from build123d import *

# Parameters (mm, degrees)
F1_DEPTH       = 15
F3_D           = 3.1
F3_DEPTH       = 15
F3_TIP         = 0.9313339595
F4_W           = 15
F4_H           = 3
F5_DEPTH       = 15
F8_D           = 3.1
F8_DEPTH       = 3
F8_TIP         = 0.9313339595
F8_ON_F7_D     = 3.1
F8_ON_F7_DEPTH = 3
F8_ON_F7_TIP   = 0.9313339595


with BuildPart() as f1:
    # F0 (on Front) → F1 (new body)
    with BuildSketch(Plane.XZ):
        with BuildLine():
            Line((-7.4164065372, 11.0490259535), (-19.4164065372, 11.0490259535))
            Line((-19.4164065372, 11.0490259535), (-19.4164065372, 8.0490259535))
            Line((-19.4164065372, 8.0490259535), (-19.4164065372, -10.7509740465))
            Line((-19.4164065372, -10.7509740465), (21.5835934628, -10.7509740465))
            Line((21.5835934628, -10.7509740465), (21.5835934628, 8.0490259535))
            Line((21.5835934628, 8.0490259535), (21.5835934628, 15.5490259535))
            Line((21.5835934628, 15.5490259535), (11.9898709467, 15.5490259535))
            ThreePointArc((11.9898709467, 15.5490259535), (1.0835934628, 23.3204583115), (-9.8226840211, 15.5490259535))
            Line((-9.8226840211, 15.5490259535), (-19.4164065372, 15.5490259535))
            Line((-19.4164065372, 15.5490259535), (-19.4164065372, 12.5490259535))
            Line((-19.4164065372, 12.5490259535), (-7.4164065372, 12.5490259535))
            ThreePointArc((-7.4164065372, 12.5490259535), (1.0835934628, 20.29968098), (9.5835934628, 12.5490259535))
            Line((9.5835934628, 12.5490259535), (15.1835934628, 12.5490259535))
            Line((15.1835934628, 12.5490259535), (15.1835934628, 11.0490259535))
            Line((15.1835934628, 11.0490259535), (12.5835934628, 11.0490259535))
            Line((12.5835934628, 11.0490259535), (9.5835934628, 11.0490259535))
            ThreePointArc((9.5835934628, 11.0490259535), (1.0835934628, 3.294835898), (-7.4164065372, 11.0490259535))
        make_face()
    extrude(amount=F1_DEPTH)

    # F3
    with Locations(Plane.XY.offset(15.5490259535)):
        with Locations((-14.6195452792, -7.5)):
            Hole(F3_D / 2, depth=F3_DEPTH)
            with Locations((0, 0, -(F3_DEPTH + F3_TIP / 2))):  # 118° drill point
                Cone(0, F3_D / 2, F3_TIP, mode=Mode.SUBTRACT)

    # F4 (on face) → F5 (join)
    with BuildSketch(Plane.XZ.offset(15)):
        with Locations((13.5835934628, -9.2509740465)):
            Rectangle(F4_W, F4_H)
        with Locations((-11.4164065372, -9.2509740465)):
            Rectangle(F4_W, F4_H)
    extrude(amount=F5_DEPTH)

    # F8
    with Locations(Plane.XY.offset(-7.7509740465)):
        with Locations((-11.4164065372, -22.5)):
            Hole(F8_D / 2, depth=F8_DEPTH)
            with Locations((0, 0, -(F8_DEPTH + F8_TIP / 2))):  # 118° drill point
                Cone(0, F8_D / 2, F8_TIP, mode=Mode.SUBTRACT)

    # F8 on F7
    with Locations(Plane.XY.offset(-7.7509740465)):
        with Locations((13.5835934628, -22.5)):
            Hole(F8_ON_F7_D / 2, depth=F8_ON_F7_DEPTH)
            with Locations((0, 0, -(F8_ON_F7_DEPTH + F8_ON_F7_TIP / 2))):  # 118° drill point
                Cone(0, F8_ON_F7_D / 2, F8_ON_F7_TIP, mode=Mode.SUBTRACT)


solid = f1.part
Here's how the part is built. I have some questions about the finished solid (model axes, mm). A direction names the side the tool comes from. Give positions to 0.01 mm unless a question says otherwise; leave off trailing zeros. Order: outer loops, then holes, each group sorted by start corner. A loop starts at its lowest first (then second) coordinate and runs counter-clockwise, first axis right, second up. Notation, with made-up numbers: M 55.25,-9.5 L 108.25,-9.5 A21 cw 108.25,18.5 Z; hole C 50,1.5 d9. An arc over 180 degrees is marked long. Answer as a JSON object with one key per item and string values. Group by question number.
1) Suppose I cut it at C-C, the plane x = -5. Write out the boundary of the cut face in (y, z).
2) Suppose I cut it at D-D, the plane y = -26.75. Write out the boundary of the cut face in (x, z), plus the area to 3 significant figures.
3) I'm going to push flat-ended pins straight in: pin 1 Ø10 at (y, z) = (-15.5, -2.5) entering from -X; pin 2 Ø8 at (x, y) = (-5.5, -9.5) entering from +Z; pin 3 Ø3.5 at (y, z) = (-23.5, -9) entering from +X; pin 4 Ø13 at (x, y) = (-12.5, -4) entering from +Z. Where does each tip first touch, or does it pass through?
4) We'd pull the mould along Y, two halves only. Please class faces 5 (the conical face through (-14.89, -7.49, -0.22)), 6 (the flat face through (0.8, -14.8, -10.751)): pulls with the +Y half, pulls with the -Y half, needs draft (parallel to the pull), parting line crosses it, or undercut.
5) Suppose I cut it at A-A, the plane z = 10. Write out the boundary of the cut face in (x, y).
6) Suppose I cut it at B-B, the plane y = -22.5. Write out the boundary of the cut face in (x, z).
7) Please list where these lines run through material, in increasing order: L1, parallel to X at y = -22.5, z = -9.45; L2, parallel to X at y = -6.25, z = 13; L3, parallel to X at y = -7.5, z = 7.75. Write a range as [from, to].
8) On a 3-axis mill with a long thin cutter (end or side, diameter ignored), from which of +Z, -Z, +X, -X, +Y, -Y can I reach the whole of each face in a straight line? I mean faces 1 (the flat face through (-18.916, -22, -9)), 2 (the flat face through (-11.5, -20.7, -7.751)), 3 (the flat face through (-3.916, -22, -9)), 4 (the flat face through (17, -7, 15.549)). Say none if no direction works.
Results found:
{
 "1": {"outline": "M -30,-10.75 L 0,-10.75 L 0,5.84 L -15,5.84 L -15,-7.75 L -30,-7.75 Z; M -15,17.75 L 0,17.75 L 0,21.59 L -15,21.59 Z"},
 "2": {"outline": "M -18.92,-10.75 L -3.92,-10.75 L -3.92,-7.75 L -18.92,-7.75 Z; M 6.08,-10.75 L 21.08,-10.75 L 21.08,-7.75 L 6.08,-7.75 Z", "area": "90.0 mm²"},
 "3": {"pin 1": "x = -19.42", "pin 2": "z = 23.03", "pin 3": "x = 21.08", "pin 4": "z = 20.89"},
 "4": {"face 5": "undercut", "face 6": "needs draft"},
 "5": {"outline": "M -19.42,-15 L -7.25,-15 L -7.25,0 L -19.42,0 Z; M 9.42,-15 L 21.58,-15 L 21.58,0 L 9.42,0 Z; hole C -14.62,-7.5 d3.1"},
 "6": {"outline": "M -18.92,-10.75 L -12.97,-10.75 L -12.97,-7.75 L -18.92,-7.75 Z; M -9.87,-10.75 L -3.92,-10.75 L -3.92,-7.75 L -9.87,-7.75 Z; M 6.08,-10.75 L 12.03,-10.75 L 12.03,-7.75 L 6.08,-7.75 Z; M 15.13,-10.75 L 21.08,-10.75 L 21.08,-7.75 L 15.13,-7.75 Z"},
 "7": {"L1": "[-18.92, -12.97], [-9.87, -3.92], [6.08, 12.03], [15.13, 21.08]", "L2": "[-19.42, -15.54], [-13.7, -7.36], [9.53, 21.58]", "L3": "[-19.42, -16.17], [-13.07, -6.41], [8.58, 21.58]"},
 "8": {"face 1": "+Z, -Z, -X, -Y", "face 2": "+Z, +X, -X, -Y", "face 3": "+Z, -Z, -Y", "face 4": "+Z, +X, +Y, -Y"}
}
